Work out the finished part from the listing and answer in its coordinate system (mm). A direction names the side the tool comes from. Round coordinates to 2 decimals unless told otherwise and drop trailing zeros. Write each loop counter-clockwise with the first axis right and the second up, starting at its lowest first coordinate (ties: lowest second). Pieces come first, ordered by that corner, then holes. Notation, with made-up numbers: M 56,-1 L 86,-1 A20 ccw 86,28 Z; hole C -33.75,69.5 d3. An arc over 180 degrees is marked long. One line per item, written item: value. Start each with the question number.
Q1. Consider probe 1 along Y at (x, z) = (0.9, -10.5); probe 2 along X at (y, z) = (8, 0.25); probe 3 along X at (y, z) = (-8.25, 5.75). Determine where each line is inside the solid, lowest interval first.
Q2. Find section C-C (z = 8). Write down the section's boundary in (x, y), and give its area (3 significant figures).
Q3. Find section D-D (y = -0.5). Write down the section's boundary in (x, z).
Q4. A tool of negligible diameter and unlimited length cuts with its end or side. For faces 1 (the flat face through (4, 0, -3)), 2 (the flat face through (1, -12, 0)), 3 (the cylindrical face through (7.493, 1.048, 0.434)), 4 (the flat face through (-1, -10, -10.5)), from which of +Z, -Z, +X, -X, +Y, -Y can it reach the whole face along a straight path? Write none if from no direction.
Q5. The mould has two halves that part along Y. Classify faces 5 (the flat face through (2, -2, 0)), 6 (the cylindrical face through (5.479, -0.905, 0.867)), 7 (the cylindrical face through (0.99, 10.99, -10.37)), 8 (the cylindrical face through (0.99, 9.01, 10.37)): released by +Y, released by -Y, zero draft, split by the parting line, or undercut.
Q6. Find section A-A (y = 10). Write down the section's boundary in (x, z).
Q7. Given pin 1 Ø0.9 at (x, z) = (-1.5, -1.5) entering from +Y; pin 2 Ø2 at (x, y) = (3.5, 5) entering from +Z; pin 3 Ø3 at (y, z) = (-2, 10.5) entering from -X, each flat-ended and moving along its own axis, determine where each tip first touches the part or whether it passes through.
Q8. Find section B-B (x = 1.5). Write down the section's boundary in (y, z).
from build123d import *

# Parameters (mm, degrees)
SKETCH1_W           = 25
SKETCH1_H           = 24
SKETCH1_R           = 1
BOSS_EXTRUDE1_DEPTH = 2
SKETCH2_W           = 8
SKETCH2_H           = 8
BOSS_EXTRUDE2_DEPTH = 2
SKETCH3_R           = 4
BOSS_EXTRUDE3_DEPTH = 3
SKETCH4_R           = 2
BOSS_EXTRUDE4_DEPTH = 1
SKETCH5_W           = 21
SKETCH5_H           = 6
BOSS_EXTRUDE5_DEPTH = 3


with BuildPart() as part:
    # Sketch1 → Boss-Extrude1 (new body)
    with BuildSketch(Plane(origin=(0, 0, 0), x_dir=(0, 0, -1), z_dir=(1, 0, 0))):
        Rectangle(SKETCH1_W, SKETCH1_H)
        with Locations((10.5, 10)):
            Circle(SKETCH1_R, mode=Mode.SUBTRACT)
        with Locations((10.5, -2)):
            Circle(SKETCH1_R, mode=Mode.SUBTRACT)
        with Locations(Location((-10.5, 10, 0), (0, 0, 180))):
            Circle(SKETCH1_R, mode=Mode.SUBTRACT)
        with Locations(Location((-10.5, -2, 0), (0, 0, 180))):
            Circle(SKETCH1_R, mode=Mode.SUBTRACT)
    extrude(amount=BOSS_EXTRUDE1_DEPTH)

    # Sketch2 → Boss-Extrude2 (add)
    with BuildSketch(Plane(origin=(2, 0, 0), x_dir=(0, 0, -1), z_dir=(1, 0, 0))):
        with Locations((0, 3)):
            Rectangle(SKETCH2_W, SKETCH2_H)
    extrude(amount=BOSS_EXTRUDE2_DEPTH)

    # Sketch3 → Boss-Extrude3 (add)
    with BuildSketch(Plane(origin=(4, 0, 0), x_dir=(0, 0, -1), z_dir=(1, 0, 0))):
        with Locations((0, 3)):
            Circle(SKETCH3_R)
    extrude(amount=BOSS_EXTRUDE3_DEPTH)

    # Sketch4 → Boss-Extrude4 (add)
    with BuildSketch(Plane(origin=(7, 0, 0), x_dir=(0, 0, -1), z_dir=(1, 0, 0))):
        with Locations((0, 3)):
            Circle(SKETCH4_R)
    extrude(amount=BOSS_EXTRUDE4_DEPTH)

    # Sketch5 → Boss-Extrude5 (add)
    with BuildSketch(Plane.ZY):
        with Locations((0, -9.5)):
            Rectangle(SKETCH5_W, SKETCH5_H)
    extrude(amount=BOSS_EXTRUDE5_DEPTH)


solid = part.part
The answers:
1. probe 1: -12 to -3, -1 to 9, 11 to 12
1. probe 2: 0 to 2
1. probe 3: -3 to 2
2. outline: M -3,-12.5 L 0,-12.5 L 0,-12 L 2,-12 L 2,12 L 0,12 L 0,-6.5 L -3,-6.5 Z
2. area: 66.0 mm2
3. outline: M 0,-12.5 L 2,-12.5 L 2,-4 L 4,-4 L 4,-1.94 L 7,-1.94 L 7,1.94 L 4,1.94 L 4,4 L 2,4 L 2,12.5 L 0,12.5 Z
4. face 1: -Z, +X, -Y
4. face 2: +Z, -Z, +X, -Y
4. face 3: +X
4. face 4: -Z, -X, +Y, -Y
5. face 5: zero draft
5. face 6: split by the parting line
5. face 7: undercut
5. face 8: undercut
6. outline: M 0,-12.5 L 2,-12.5 L 2,-11.5 L 0,-11.5 Z; M 0,-9.5 L 2,-9.5 L 2,9.5 L 0,9.5 Z; M 0,11.5 L 2,11.5 L 2,12.5 L 0,12.5 Z
7. pin 1: y = -6.5
7. pin 2: z = 4
7. pin 3: x = 0
8. outline: M -12,-12.5 L 12,-12.5 L 12,12.5 L -12,12.5 Z; hole C -2,-10.5 d2; hole C -2,10.5 d2; hole C 10,-10.5 d2; hole C 10,10.5 d2
